```python
from build123d import *

# Parameters (mm, degrees)
TOP_PLATE_DIAMETER_R           = 73.025
TOP_PLATE_EXTRUDE_DEPTH        = 12.7
FUEL_PORT_CLEARANCE_DIAMETER_R = 14.2875
FUEL_PORT_CLEARANCE_HOLE_DEPTH = 13.7
ASSEMBLY_BOLT_DIAMETER_R       = 3.571875
ASSEMBLY_BOLT_DEPTH            = 12.7
CIRPATTERN1_COUNT              = 12
LOX_PORT_REACH                 = 14.7
SKETCH7_R                      = 8.7122


with BuildPart() as part:
    # Top Plate Diameter → Top Plate Extrude (new body)
    with BuildSketch(Plane(origin=(0, 0, 0), x_dir=(1, 0, 0), z_dir=(0, 1, 0))):
        Circle(TOP_PLATE_DIAMETER_R)
    extrude(amount=TOP_PLATE_EXTRUDE_DEPTH)

    # Fuel Port Clearance Diameter → Fuel Port Clearance Hole (cut, through all)
    with BuildSketch(Plane(origin=(0, 12.7, 0), x_dir=(1, 0, 0), z_dir=(0, 1, 0))):
        Circle(FUEL_PORT_CLEARANCE_DIAMETER_R)
    extrude(amount=-FUEL_PORT_CLEARANCE_HOLE_DEPTH, mode=Mode.SUBTRACT)

    # Assembly Bolt Diameter → Assembly Bolt (cut)
    with BuildSketch(Plane(origin=(0, 12.7, 0), x_dir=(1, 0, 0), z_dir=(0, 1, 0))):
        with Locations((-58.882838371, 15.777608989)):
            Circle(ASSEMBLY_BOLT_DIAMETER_R)
    assembly_bolt = extrude(amount=-ASSEMBLY_BOLT_DEPTH, mode=Mode.SUBTRACT)

    # CirPattern1: Assembly Bolt ×12 about axis
    cirpattern1_axis = Axis((0, 0, 0), (0, 1, 0))
    for i in range(1, CIRPATTERN1_COUNT):
        add(assembly_bolt.rotate(cirpattern1_axis, i * 360 / CIRPATTERN1_COUNT), mode=Mode.SUBTRACT)

    # Sketch7 → LOX Port (cut, up to next)
    with BuildSketch(Plane(origin=(0, 12.7, 0), x_dir=(1, 0, 0), z_dir=(0, 1, 0)), mode=Mode.PRIVATE) as lox_port_sk1:
        with Locations((-30.226, 0)):
            Circle(SKETCH7_R)
    lox_port_tool1 = extrude(lox_port_sk1.sketch, amount=-LOX_PORT_REACH, mode=Mode.PRIVATE) & part.part
    add(lox_port_tool1.solids().sort_by_distance((-30.226, 12.7, 0))[0], mode=Mode.SUBTRACT)

    # Sketch9 → Cut-Revolve1 (revolve, cut)
    with BuildSketch(Plane.XY):
        with BuildLine():
            Line((-41.3385, 12.7), (-39.9923, 11.922771068))
            Line((-39.9923, 11.922771068), (-39.9923, 10.3124))
            ThreePointArc((-39.9923, 10.3124), (-39.953630803, 10.117996816), (-39.843510245, 9.953189755))
            Line((-39.843510245, 9.953189755), (-38.9382, 9.04787951))
            Line((-38.9382, 9.04787951), (-38.9382, 12.7))
            Line((-38.9382, 12.7), (-41.3385, 12.7))
        make_face()
    revolve(axis=Axis((-30.226, -7.468881995, 0), (0, 1, 0)), mode=Mode.SUBTRACT)


solid = part.part
```
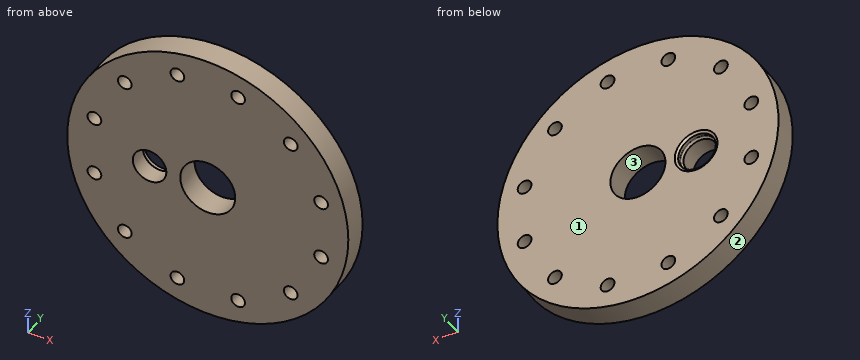
Input: part model. Units: mm. Frame: model coordinates. Face numbers are marked on the shaded views. Coordinates: 2 decimals unless noted, no trailing zeros. Write each loop counter-clockwise with the first axis right and the second up, starting at its lowest first coordinate (ties: lowest second). Pieces come first, ordered by that corner, then holes. Notation, with made-up numbers: (55.5, 60.25) -> (90.5, 60.25) arc R8 ccw to (90.5, 70.25) -> close; hole circle Ø11 at (3.5, 25.25). An arc over 180 degrees is marked (long way). Write each question's results on one line, items separated by ' | '.
Item 1: Mould query, pull axis Z, two halves, no side actions, for the marked faces 1, 2 and 3. Classes: +Z half, -Z half, draft (parallel to the pull), parting line (faces both ways), or undercut.
Conclusion:
face 1: draft | face 2: parting line | face 3: undercut
Item 2: Pin query (flat end, axial travel): pin 1 Ø1.5 at (x, y) = (-17, 3) entering from -Z; pin 2 Ø11.5 at (x, z) = (43.11, 43.11) entering from +Y; pin 3 Ø2 at (x, y) = (-45, 8) entering from +Z; pin 4 Ø1.5 at (y, z) = (11, 5) entering from +X. Return the tip coordinate at first contact, or that it passes through.
Conclusion:
pin 1: stops at z = -71.19 | pin 2: stops at y = 12.7 | pin 3: stops at z = 58.28 | pin 4: stops at x = 72.9
Item 3: Section query D-D on z = -25.5. Return loops of the section in (x, y), plus the area to 3 significant figures.
Conclusion:
outline: (-68.43, 0) -> (68.43, 0) -> (68.43, 12.7) -> (-68.43, 12.7) -> close | area: 1,740 mm^2
Item 4: Section query B-B on z = 0. Count the separate pieces of the cut face and the enclosed holes in it, plus the area to 3 significant figures.
Conclusion:
separate pieces: 3 | enclosed holes: 0 | area: 1,260 mm^2
Item 5: Material intervals for probe 1 along X at (y, z) = (7, 14.5); probe 2 along Z at (x, y) = (-60, 8), sorted ascending.
Conclusion:
probe 1: x = -71.57 to -62.22, -55.55 to 55.55, 62.22 to 71.57 | probe 2: z = -41.63 to -19.17, -12.38 to 12.38, 19.17 to 41.63
Item 6: Section query A-A on x = 0. Return loops of the section in (y, z) (1 decimal), plus the area to 3 significant figures.
Conclusion:
outline: (0, -73) -> (12.7, -73) -> (12.7, -14.3) -> (0, -14.3) -> close; (0, 14.3) -> (12.7, 14.3) -> (12.7, 73) -> (0, 73) -> close | area: 1,490 mm^2
